Check sheet for the drawn part. Datum: minimum x, y, z corner. Units: mm. A direction names the side the tool comes from. Coordinates: 2 decimals unless noted, no trailing zeros. Write each loop counter-clockwise with the first axis right and the second up, starting at its lowest first coordinate (ties: lowest second). Pieces come first, ordered by that corner, then holes. Notation, with made-up numbers: (-27, 55.25) -> (23, 55.25) arc R11 cw to (23, 75.25) -> close; hole circle Ø6 at (-13, -10.5). An arc over 180 degrees is marked (long way). Answer in a Markdown table with one row per item. Add a question column.
1. Cross-section at C-C on z = 210.5. Record the cut outline in (x, y).
2. Depth check by flat-ended pin: P1, Ø4, axis at x = 81, z = 104.5, coming from the +Y side; P2, Ø12, axis at x = 64.5, z = 77.5, coming from the +Y side; P3, Ø12, axis at y = 182.5, z = 47, coming from the -X side. Enter the tip coordinate at first touch or a pass-through.
3. Set-up check for the marked faces 1, 2 and 3: record each of +Z, -Z, +X, -X, +Y, -Y from which the full face is reachable in a straight line by a thin tool's end or side.
4. Cross-section at B-B on x = 17.5. Record the cut outline in (y, z).
5. Cross-section at A-A on y = 154.5. Record the cut outline in (x, z), and give its area (3 significant figures).
6. Scan lines: L1, parallel to Y at x = 125.5, z = 147.5; L2, parallel to Z at x = 222, y = 89. Record each from-to range of solid material in increasing order. Write a range as from..to.
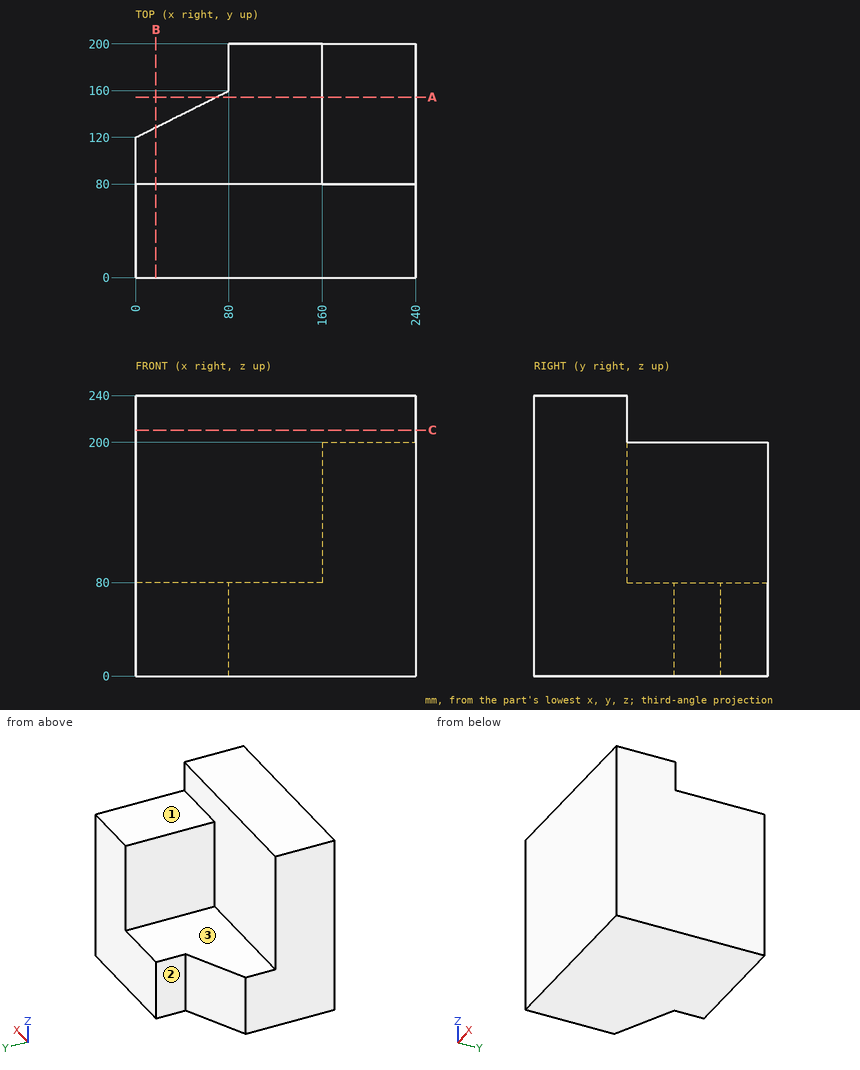
Results found:
| question | item | result |
|---|---|---|
| 1 | outline | (0, 0) -> (240, 0) -> (240, 80) -> (0, 80) -> close |
| 2 | P1 | stops at y = 80 |
| 2 | P2 | stops at y = 155.25 |
| 2 | P3 | stops at x = 80 |
| 3 | face 1 | +Z, +X, -X, +Y |
| 3 | face 2 | +Z, -Z, -X, +Y |
| 3 | face 3 | +Z, -X, +Y |
| 4 | outline | (0, 0) -> (128.75, 0) -> (128.75, 80) -> (80, 80) -> (80, 240) -> (0, 240) -> close |
| 5 | outline | (69, 0) -> (240, 0) -> (240, 200) -> (160, 200) -> (160, 80) -> (69, 80) -> close |
| 5 | area | 23,300 mm^2 |
| 6 | L1 | y = 0..80 |
| 6 | L2 | z = 0..200 |
